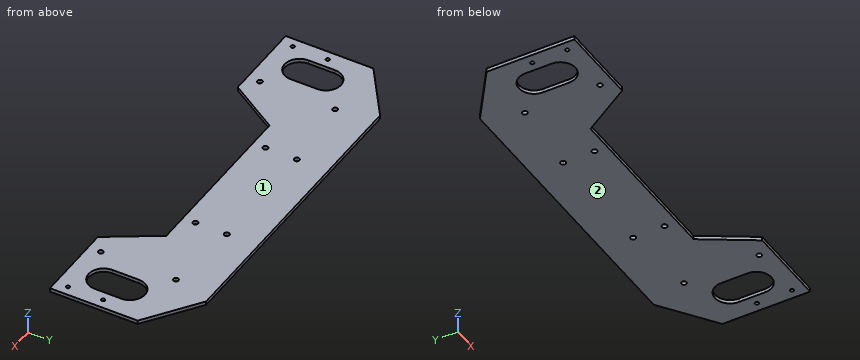
```python
from build123d import *

# Parameters (mm, degrees)
SKETCH_1_W                  = 320
SKETCH_1_H                  = 100
EXTRUDE_1_DEPTH             = 3
HOLE_WIZARD_4_0_4_1_D       = 4
HOLE_WIZARD_4_2_4_2_1_D     = 4.2
PATTERN_LINEAR_1_COUNT      = 2
PATTERN_LINEAR_1_PITCH      = 95
PATTERN_LINEAR_1_COUNT_DIR2 = 2
PATTERN_LINEAR_1_PITCH_DIR2 = 25
CUT_EXTRUDE_1_DEPTH         = 3
SKETCH_8_W                  = 24
SKETCH_8_H                  = 45
CUT_EXTRUDE_6_DEPTH         = 3
PATTERN_LINEAR_2_COUNT      = 2
PATTERN_LINEAR_2_PITCH      = 60
PATTERN_LINEAR_2_COPY_1_D   = 4
HOLE_WIZARD_3_0_3_1_D       = 3
CUT_EXTRUDE_8_DEPTH         = 3
FILLET_1_R                  = 12


with BuildPart() as part:
    # 草图1 → 凸台-拉伸1 (new body)
    with BuildSketch(Plane.XY):
        Rectangle(SKETCH_1_W, SKETCH_1_H)
    extrude(amount=EXTRUDE_1_DEPTH)

    # Ø4.0 (4) 直径孔1 (through all)
    with Locations(Plane(origin=(0, 0, 0), x_dir=(-1, 0, 0), z_dir=(0, 0, -1))):
        with Locations((108, -40)):
            hole_wizard_4_0_4_1 = Hole(HOLE_WIZARD_4_0_4_1_D / 2)

    # 镜向1: Ø4.0 (4) 直径孔1 across plane
    add(hole_wizard_4_0_4_1.mirror(Plane(origin=(0, 0, 0), x_dir=(0, 0, 1), z_dir=(1, 0, 0))), mode=Mode.SUBTRACT)

    # Ø4.2 (4.2) 直径孔1 (through all)
    with Locations(Plane(origin=(0, 0, 0), x_dir=(-1, 0, 0), z_dir=(0, 0, -1))):
        with Locations((47.5, 0)):
            hole_wizard_4_2_4_2_1 = Hole(HOLE_WIZARD_4_2_4_2_1_D / 2)

    # 阵列(线性)1: Hole Wizard 4.2 _4.2_ _1 2 × 2
    with Locations(*[(i * PATTERN_LINEAR_1_PITCH, j * PATTERN_LINEAR_1_PITCH_DIR2, 0) for i in range(PATTERN_LINEAR_1_COUNT) for j in range(PATTERN_LINEAR_1_COUNT_DIR2) if (i, j) != (0, 0)]):
        add(hole_wizard_4_2_4_2_1, mode=Mode.SUBTRACT)

    # 草图6 → 切除-拉伸1 (cut)
    with BuildSketch(Plane(origin=(0, 0, 0), x_dir=(-1, 0, 0), z_dir=(0, 0, -1))):
        Polygon((0, -50), (0, -10), (70, -10), (95, -50), align=None)
    cut_extrude_1 = extrude(amount=-CUT_EXTRUDE_1_DEPTH, mode=Mode.SUBTRACT)

    # 镜向2: 切除-拉伸1 across plane
    add(cut_extrude_1.mirror(Plane(origin=(0, -50, 3), x_dir=(0, 0, 1), z_dir=(1, 0, 0))), mode=Mode.SUBTRACT)

    # 草图8 → 切除-拉伸6 (cut)
    with BuildSketch(Plane(origin=(0, 0, 0), x_dir=(-1, 0, 0), z_dir=(0, 0, -1))):
        with Locations((-133, -12.5)):
            Rectangle(SKETCH_8_W, SKETCH_8_H)
    cut_extrude_6 = extrude(amount=-CUT_EXTRUDE_6_DEPTH, mode=Mode.SUBTRACT)

    # 镜向4: 切除-拉伸6 across plane
    add(cut_extrude_6.mirror(Plane(origin=(0, 0, 0), x_dir=(0, 0, 1), z_dir=(1, 0, 0))), mode=Mode.SUBTRACT)

    # 阵列(线性)2: Ø4.0 (4) 直径孔1 ×2
    with Locations(*[(0, i * PATTERN_LINEAR_2_PITCH, 0) for i in range(1, PATTERN_LINEAR_2_COUNT)]):
        add(hole_wizard_4_0_4_1, mode=Mode.SUBTRACT)

    # 阵列(线性)2 copy 1 (through all)
    with Locations(Plane(origin=(0, 60, 0), x_dir=(1, 0, 0), z_dir=(0, 0, -1))):
        with Locations((108, 40)):
            Hole(PATTERN_LINEAR_2_COPY_1_D / 2)

    # Ø3.0 (3) 直径孔1 (through all)
    with Locations(Plane.XY.offset(3)):
        with Locations((-152.5, -40), (-152.5, -12)):
            hole_wizard_3_0_3_1 = Hole(HOLE_WIZARD_3_0_3_1_D / 2)

    # 草图11 → 切除-拉伸8 (cut)
    with BuildSketch(Plane.XY.offset(3)):
        Polygon((-118, 50), (-160, 50), (-160, 20), align=None)
    cut_extrude_8 = extrude(amount=-CUT_EXTRUDE_8_DEPTH, mode=Mode.SUBTRACT)

    # 镜向6: 切除-拉伸8 across plane
    add(cut_extrude_8.mirror(Plane(origin=(0, 0, 0), x_dir=(0, 0, 1), z_dir=(1, 0, 0))), mode=Mode.SUBTRACT)

    # 镜向7: Ø3.0 (3) 直径孔1 across plane
    add(hole_wizard_3_0_3_1.mirror(Plane(origin=(0, 0, 0), x_dir=(0, 0, 1), z_dir=(1, 0, 0))), mode=Mode.SUBTRACT)

    # 圆角1
    fillet_1_edges = [part.edges().sort_by_distance(p)[0] for p in [
        (145, -35, 1.5),
        (121, -35, 1.5),
        (145, 10, 1.5),
        (121, 10, 1.5),
        (-145, -35, 1.5),
        (-121, -35, 1.5),
        (-145, 10, 1.5),
        (-121, 10, 1.5),
    ]]
    fillet(fillet_1_edges, radius=FILLET_1_R - 0.0001)  # a hair under: the kernel refuses the full size


solid = part.part
```
CAD build for the part. Positions are in the model's coordinates, mm. Face numbers are marked on the shaded views. Round coordinates to 2 decimals unless told otherwise and drop trailing zeros. Write each loop counter-clockwise with the first axis right and the second up, starting at its lowest first coordinate (ties: lowest second). Pieces come first, ordered by that corner, then holes. Notation, with made-up numbers: (40.25, -31) -> (66.25, -31) arc R18 ccw to (66.25, -25) -> close; hole circle Ø11 at (-34, 57.5). An arc over 180 degrees is marked (long way). Answer in a Markdown table with one row per item. Add a question column.
Item 1: Saw through at A-A, the plane x = -124. Write the cut outline in (y, z), then the cut area to 3 significant figures.
Item 2: Drill centre lines: line 1 (Y direction, x = 47.5, z = 0.85); line 2 (X direction, y = -4, z = 0.8); line 3 (Y direction, x = -108, z = 1.65). Where is each one in solid material? Low to high. Write a range as from..to.
Item 3: Saw through at D-D, the plane x = -81. Write the cut outline in (y, z).
Item 4: Mould opens along Z. For the marked faces 1 and 2 say: pulls with the +Z half, pulls with the -Z half, needs draft (parallel to the pull), parting line crosses it, or undercut.
Item 5: Saw through at C-C, the plane z = 0.95. Count the separate pieces of the cut face and the enclosed holes in it, then the cut area to 3 significant figures.
Item 6: Drop flat-ended pins along their axis: pin 1 Ø4.5 at (x, y) = (108, 20) entering from -Z; pin 2 Ø1.5 at (x, z) = (22.5, 1.5) entering from -Y; pin 3 Ø1.5 at (x, z) = (88.5, 1) entering from -Y. Give the stop position or say it passes through.
Item 7: Saw through at B-B, the plane y = 6.5. Write the cut outline in (x, z), then the cut area to 3 significant figures.
Findings below:
| question | item | result |
|---|---|---|
| 1 | outline | (-50, 0) -> (-30.94, 0) -> (-30.94, 3) -> (-50, 3) -> close; (5.94, 0) -> (45.71, 0) -> (45.71, 3) -> (5.94, 3) -> close |
| 1 | area | 177 mm^2 |
| 2 | line 1 | y = -10..-2.1, 2.1..22.9, 27.1..50 |
| 2 | line 2 | x = -160..-145, -121..121, 145..160 |
| 2 | line 3 | y = -50..-42, -38..18, 22..50 |
| 3 | outline | (-27.6, 0) -> (50, 0) -> (50, 3) -> (-27.6, 3) -> close |
| 4 | face 1 | pulls with the +Z half |
| 4 | face 2 | pulls with the -Z half |
| 5 | separate pieces | 1 |
| 5 | enclosed holes | 14 |
| 5 | area | 22,100 mm^2 |
| 6 | pin 1 | stops at z = 0 |
| 6 | pin 2 | stops at y = -10 |
| 6 | pin 3 | stops at y = -40.8 |
| 7 | outline | (-160, 0) -> (-141.47, 0) -> (-141.47, 3) -> (-160, 3) -> close; (-124.53, 0) -> (124.53, 0) -> (124.53, 3) -> (-124.53, 3) -> close; (141.47, 0) -> (160, 0) -> (160, 3) -> (141.47, 3) -> close |
| 7 | area | 858 mm^2 |
